Verification items for the finished model (mm, model axes). Face numbers are marked on the shaded views. A direction names the side the tool comes from. Round coordinates to 2 decimals unless told otherwise and drop trailing zeros. Write each loop counter-clockwise with the first axis right and the second up, starting at its lowest first coordinate (ties: lowest second). Pieces come first, ordered by that corner, then holes. Notation, with made-up numbers: M 81.25,37.25 L 111.25,37.25 A21 cw 111.25,68.25 Z; hole C 71,-11 d7. An arc over 180 degrees is marked long. One line per question, with ' | ' between items. Start each with the question number.
Q1. Gauge pin test, flat ends, axial feed: pin 1 (21.5 mm diameter, centred on x = -26, y = -27.5, fed in from +Z); pin 2 (7.5 mm diameter, centred on x = -30, z = 25, fed in from -Y); pin 3 (10 mm diameter, centred on y = -41.5, z = 5, fed in from +X). Record the tip position at first contact, or that the pin passes through.
Q2. Tool access check on the marked faces 4, 5, 6 and 7. Record the directions out of +Z, -Z, +X, -X, +Y, -Y that give a thin tool (end or side, any length) a straight path to the whole face; none if there is none.
Q3. Cross-section at A-A (z = 10.5). Record the boundary of the cut face in (x, y), then the cut area to 3 significant figures.
Q4. Cross-section at B-B (y = -57.15). Record the boundary of the cut face in (x, z), then the cut area to 3 significant figures.
Q5. Cross-section at D-D (z = 28). Record the boundary of the cut face in (x, y), then the cut area to 3 significant figures.
Q6. Thickness scan on line 1 along Y through (x, z) = (-34, 9); line 2 along X through (y, z) = (-10, 25); line 3 along Y through (x, z) = (-33, 16.5). Record the ranges inside material, lowest first. Write a range as from..to.
Q7. Release check for a two-part mould opening along X. For the marked faces 1, 2 and 3 record: released by +X, released by -X, zero draft, split by the parting line, or undercut.
Q8. Cross-section at C-C (x = -39.5). Record the boundary of the cut face in (y, z), then the cut area to 3 significant figures.
from build123d import *

# Parameters (mm, degrees)
F0_W      = 50.8
F0_H      = 12.7
F1_DEPTH  = 38.1
F2_W      = 25.4
F2_H      = 23.9464748895
F3_DEPTH  = 12.7
F5_DEPTH  = 12.7
F6_DEPTH  = 25.4
F7_DEPTH  = 6.35
F8_R      = 6.35
F9_DEPTH  = 25.4
F10_R     = 6.35
F11_DEPTH = 25.4
F12_R     = 3.0660512242


with BuildPart() as f1:
    # F0 (on Top) → F1 (new body)
    with BuildSketch(Plane.XY):
        with Locations((-34.4613061011, -6.35)):
            Rectangle(F0_W, F0_H)
    extrude(amount=F1_DEPTH)

    # F2 (on face) → F3 (join)
    with BuildSketch(Plane(origin=(0, 0, 0), x_dir=(1, 0, 0), z_dir=(0, 0, -1))):
        with BuildLine():
            ThreePointArc((-47.1613061011, 25.4), (-50.88104998, 16.4197438789), (-59.8613061011, 12.7))
            Line((-59.8613061011, 12.7), (-9.0613061011, 12.7))
            ThreePointArc((-9.0613061011, 12.7), (-18.0415622222, 16.4197438789), (-21.7613061011, 25.4))
            Line((-21.7613061011, 25.4), (-47.1613061011, 25.4))
        make_face()
        with Locations((-34.4613061011, 37.3732374447)):
            Rectangle(F2_W, F2_H)
    extrude(amount=-F3_DEPTH)

    # F4 (on face) → F5 (join)
    with BuildSketch(Plane.XY.offset(12.7)):
        with BuildLine():
            Line((-44.4810364292, -49.3464748895), (-24.4415757729, -49.3464748895))
            ThreePointArc((-24.4415757729, -49.3464748895), (-34.4613061011, -44.45), (-44.4810364292, -49.3464748895))
        make_face()
        with BuildLine():
            ThreePointArc((-44.4810364292, -49.3464748895), (-38.5868015157, -69.1612567029), (-21.7613061011, -57.15))
            ThreePointArc((-21.7613061011, -57.15), (-22.4500493981, -53.0245045854), (-24.4415757729, -49.3464748895))
            Line((-24.4415757729, -49.3464748895), (-44.4810364292, -49.3464748895))
        make_face()
    extrude(amount=F5_DEPTH)

    # F6 (add): a face of the model
    f6_faces = [f1.faces().sort_by_distance(p)[0] for p in [
        (-34.4613061011, -57.15, 25.4),
    ]]
    extrude(f6_faces, amount=-F6_DEPTH)

    # F7 (add): faces of the model
    f7_faces = [f1.faces().sort_by_distance(p)[0] for p in [
        (-45.8211712652, -49.3464748895, 6.35),
        (-23.101440937, -49.3464748895, 6.35),
    ]]
    extrude(f7_faces, amount=F7_DEPTH)

    # F8 (on face) → F9 (cut)
    with BuildSketch(Plane.XY.offset(25.4)):
        with Locations((-34.4613061011, -57.15)):
            Circle(F8_R)
    extrude(amount=-F9_DEPTH, mode=Mode.SUBTRACT)

    # F10 (on face) → F11 (cut)
    with BuildSketch(Plane.XZ.offset(12.7)):
        with Locations((-34.4613061011, 25.4)):
            Circle(F10_R)
    extrude(amount=-F11_DEPTH, mode=Mode.SUBTRACT)

    # F12
    f12_edges = [f1.edges().sort_by_distance(p)[0] for p in [
        (-59.861306, -6.35, 38.1),
        (-9.061306, -6.35, 38.1),
    ]]
    fillet(f12_edges, radius=F12_R)


solid = f1.part
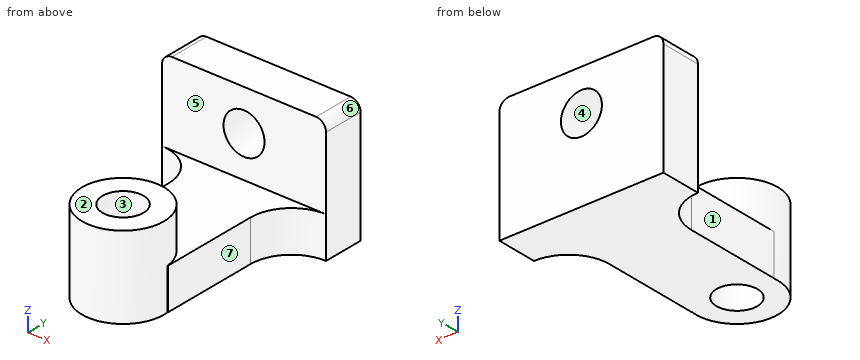
Determined:
1) pin 1: stops at z = 12.7 | pin 2: stops at y = -69.83 | pin 3: stops at x = -21.76
2) face 4: +Y | face 5: +Z, +X, -X | face 6: +Z, +X, +Y, -Y | face 7: +Z, -Z, +X, -Y
3) outline: M -59.86,-12.7 A12.7 cw -47.16,-25.4 L -47.16,-55.7 L -47.08,-55.7 A12.7 ccw long -21.84,-55.7 L -21.76,-55.7 L -21.76,-25.4 A12.7 cw -9.06,-12.7 L -9.06,0 L -59.86,0 Z; hole C -34.46,-57.15 d12.7 | area: 1,970 mm²
4) outline: M -47.16,0 L -40.81,0 L -40.81,25.4 L -47.16,25.4 Z; M -28.11,0 L -21.76,0 L -21.76,25.4 L -28.11,25.4 Z | area: 323 mm²
5) outline: M -59.86,-12.7 L -40.25,-12.7 L -40.25,0 L -59.86,0 Z; M -28.67,-12.7 L -9.06,-12.7 L -9.06,0 L -28.67,0 Z | area: 498 mm²
6) line 1: y = -69.84..-63.48, -50.82..0 | line 2: x = -59.86..-40.8, -28.12..-9.06 | line 3: y = -69.77..-63.33, -50.97..-44.53, -12.7..0
7) face 1: released by -X | face 2: zero draft | face 3: undercut
8) outline: M -68.81,0 L -61.01,0 L -61.01,25.4 L -68.81,25.4 Z; M -53.29,0 L 0,0 L 0,21.54 L -12.7,21.54 L -12.7,12.7 L -45.49,12.7 L -45.49,25.4 L -53.29,25.4 Z; M -12.7,29.26 L 0,29.26 L 0,38.1 L -12.7,38.1 Z | area: 1,200 mm²
